Could you check a few things on this drawing? It's one solid part, dimensions in mm from its lowest x, y, z. A direction names the side the tool comes from. Give positions to 0.01 mm unless a question says otherwise; leave off trailing zeros. Order: outer loops, then holes, each group sorted by start corner. A loop starts at its lowest first (then second) coordinate and runs counter-clockwise, first axis right, second up.
Item 1: Which directions (+Z, -Z, +X, -X, +Y, -Y) give clear straight access to the entire face, cutting with the end or side of a thin tool? Please do the marked faces 5 and 6.
Item 2: I'm going to push flat-ended pins straight in: pin 1 Ø3.5 at (x, y) = (4, 51) entering from -Z; pin 2 Ø4 at (x, z) = (4.5, 8) entering from +Y; pin 3 Ø2.5 at (x, y) = (4, 51) entering from -Z; pin 4 Ø2 at (x, z) = (4, 16.5) entering from -Y. Where does each tip first touch, or does it pass through?
Item 3: If we mould it in two halves opening along Z, with no side actions, what happens to the marked faces 1, 2, 3 and 4? For each: +Z half, -Z half, draft (parallel to the pull), parting line (faces both ways), or undercut.
Item 4: I want a section at A-A, the plane y = 51. Write out the boundary of the cut face in (x, z).
Item 5: I want a section at C-C, the plane z = 18.5. Write out the boundary of the cut face in (x, y).
Item 6: If I drill on line 1 along Z through (x, y) = (4, 7.5); line 2 along Y through (x, z) = (4, 20.2); line 3 along X through (y, z) = (33, 9.5), over which ranges is the centre line in solid material (lowest first)?
Item 7: I want a section at B-B, the plane x = 6.75. Write out the boundary of the cut face in (y, z).
Item 8: I want a section at D-D, the plane y = 33. Write out the boundary of the cut face in (x, z).
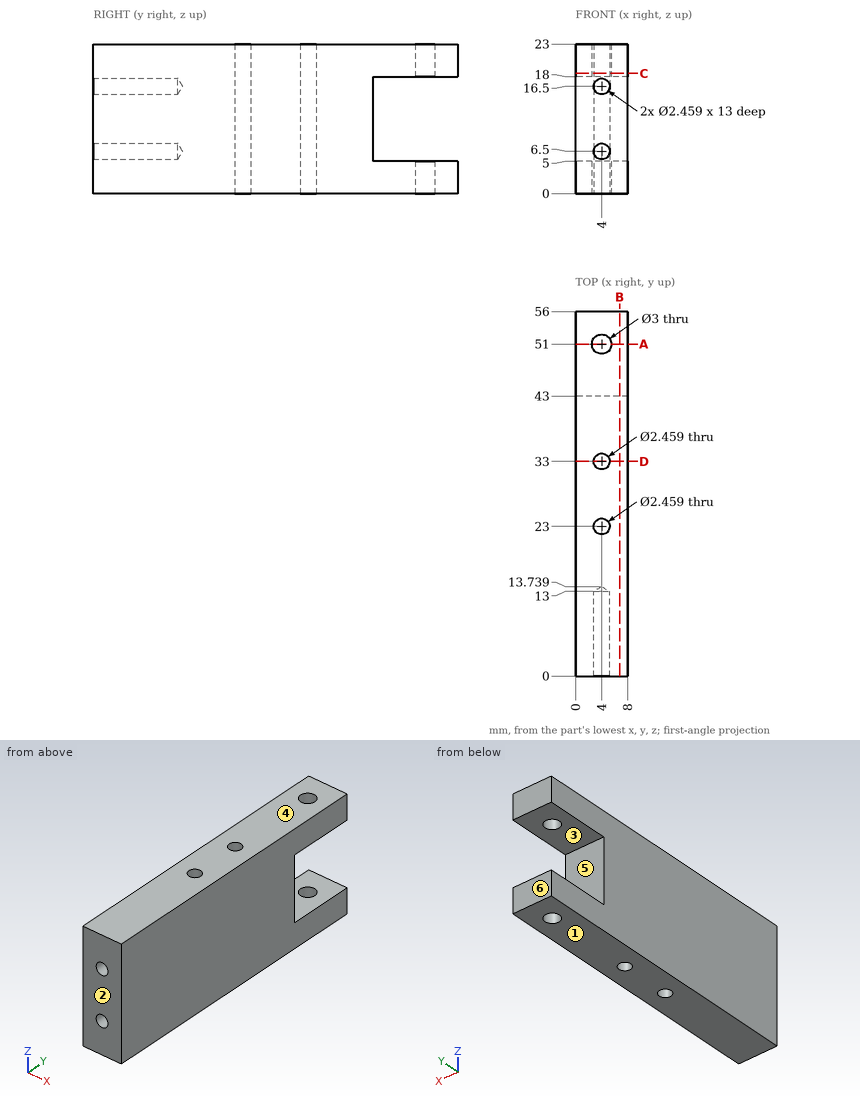
Results list:
1. face 5: +X, -X, +Y
1. face 6: +Z, -Z, +X, -X, +Y
2. pin 1: stops at z = 0
2. pin 2: stops at y = 43
2. pin 3: passes through
2. pin 4: stops at y = 13.14
3. face 1: -Z half
3. face 2: draft
3. face 3: undercut
3. face 4: +Z half
4. outline: (0, 0) - (2.5, 0) - (2.5, 5) - (0, 5) - close; (0, 18) - (2.5, 18) - (2.5, 23) - (0, 23) - close; (5.5, 0) - (8, 0) - (8, 5) - (5.5, 5) - close; (5.5, 18) - (8, 18) - (8, 23) - (5.5, 23) - close
5. outline: (0, 0) - (8, 0) - (8, 56) - (0, 56) - close; hole circle Ø3 at (4, 51); hole circle Ø2.46 at (4, 23); hole circle Ø2.46 at (4, 33)
6. line 1: z = 0 to 5.27, 7.73 to 15.27, 17.73 to 23
6. line 2: y = 0 to 21.77, 24.23 to 31.77, 34.23 to 49.5, 52.5 to 56
6. line 3: x = 0 to 2.77, 5.23 to 8
7. outline: (0, 0) - (56, 0) - (56, 5) - (43, 5) - (43, 18) - (56, 18) - (56, 23) - (0, 23) - close
8. outline: (0, 0) - (2.77, 0) - (2.77, 23) - (0, 23) - close; (5.23, 0) - (8, 0) - (8, 23) - (5.23, 23) - close
